Could you check a few things on this model? Use its own coordinates, in mm. Give positions to 0.01 mm unless a question says otherwise; leave off trailing zeros. Write each loop counter-clockwise with the first axis right and the second up, starting at its lowest first coordinate (ties: lowest second). Pieces come first, ordered by that corner, then holes. Notation, with made-up numbers: (16.5, 24) - (31.5, 24) arc R25 cw to (31.5, 61) - close; hole circle Ø10 at (-9, -27.5). An arc over 180 degrees is marked (long way). Answer as CSV lines item,"result". Start each with the question number.
Q1. Imagine slicing it at D-D on z = 0.3. List the corners of the cut face in (x, y) for me, and give its area (3 significant figures).
Q2. Will these pins go through, and if not, where does the flat tip stop? pin 1 Ø3 at (x, y) = (44, 23.5) entering from +Z; pin 2 Ø2 at (x, y) = (-44, -23.5) entering from -Z.
Q3. Imagine slicing it at C-C on y = 15.5. List the corners of the cut face in (x, z) for me.
Q4. We'd pull the mould along X, two halves only. Please class faces 1 (the face through (44.65, 22.26, 0.99)), 2 (the face through (-1, 0, 0)), 3 (the face through (25.005, 11.72, 1.014)): pulls with the +X half, pulls with the -X half, needs draft (parallel to the pull), parting line crosses it, or undercut.
Q5. Imagine slicing it at A-A on x = 30. List the corners of the cut face in (y, z) for me.
Q6. If I drill on line 1 along Y through (x, z) = (44, 0.85); line 2 along Y through (x, z) = (30, 0.95); line 3 along X through (y, z) = (-10, 1.15), over which ranges is the centre line in solid material (lowest first)?
Q7. Imagine slicing it at B-B on x = 44. List the corners of the cut face in (y, z) for me.
```python
from build123d import *

# Parameters (mm, degrees)
SKETCH_W     = 94
SKETCH_H     = 53
SKETCH_R     = 1.4
PAD_DEPTH    = 2
FILLET_R     = 1
SKETCH001_R  = 5
POCKET_DEPTH = 5


with BuildPart() as part:
    # Sketch → Pad (new body)
    with BuildSketch(Plane.XY):
        Rectangle(SKETCH_W, SKETCH_H)
        with Locations((-44, 23.5)):
            Circle(SKETCH_R, mode=Mode.SUBTRACT)
        with Locations((44, 23.5)):
            Circle(SKETCH_R, mode=Mode.SUBTRACT)
        with Locations((44, -23.5)):
            Circle(SKETCH_R, mode=Mode.SUBTRACT)
        with Locations((-44, -23.5)):
            Circle(SKETCH_R, mode=Mode.SUBTRACT)
    extrude(amount=PAD_DEPTH)

    # Fillet
    fillet_edges = [part.edges().sort_by_distance(p)[0] for p in [
        (47, 0, 2),
        (47, 26.5, 1),
        (47, -26.5, 1),
        (0, -26.5, 2),
        (0, 26.5, 2),
        (-47, 0, 2),
        (-47, 26.5, 1),
        (-47, -26.5, 1),
    ]]
    fillet(fillet_edges, radius=FILLET_R)

    # Sketch001 (on Face17 of Fillet) → Pocket (cut)
    with BuildSketch(Plane.XY.offset(2)):
        with Locations((30, 11.5)):
            Circle(SKETCH001_R)
    extrude(amount=-POCKET_DEPTH, mode=Mode.SUBTRACT)


solid = part.part
```
Conclusion:
1,outline,"(-47, -25.5) arc R1 ccw to (-46, -26.5) - (46, -26.5) arc R1 ccw to (47, -25.5) - (47, 25.5) arc R1 ccw to (46, 26.5) - (-46, 26.5) arc R1 ccw to (-47, 25.5) - close; hole circle Ø2.8 at (-44, -23.5); hole circle Ø2.8 at (-44, 23.5); hole circle Ø10 at (30, 11.5); hole circle Ø2.8 at (44, -23.5); hole circle Ø2.8 at (44, 23.5)"
1,area,"4,880 mm^2"
2,pin 1,"z = 2"
2,pin 2,"through"
3,outline,"(-47, 0) - (27, 0) - (27, 2) - (-46, 2) arc R1 ccw to (-47, 1) - close; (33, 0) - (47, 0) - (47, 1) arc R1 ccw to (46, 2) - (33, 2) - close"
4,face 1,"undercut"
4,face 2,"needs draft"
4,face 3,"undercut"
5,outline,"(-26.5, 0) - (6.5, 0) - (6.5, 2) - (-25.5, 2) arc R1 ccw to (-26.5, 1) - close; (16.5, 0) - (26.5, 0) - (26.5, 1) arc R1 ccw to (25.5, 2) - (16.5, 2) - close"
6,line 1,"-26.5 to -24.9, -22.1 to 22.1, 24.9 to 26.5"
6,line 2,"-26.5 to 6.5, 16.5 to 26.5"
6,line 3,"-46.99 to 46.99"
7,outline,"(-26.5, 0) - (-24.9, 0) - (-24.9, 2) - (-25.5, 2) arc R1 ccw to (-26.5, 1) - close; (-22.1, 0) - (22.1, 0) - (22.1, 2) - (-22.1, 2) - close; (24.9, 0) - (26.5, 0) - (26.5, 1) arc R1 ccw to (25.5, 2) - (24.9, 2) - close"
